Autodesk Inventor part; units mm, degrees
ref_plane "Work Plane2" through (0, 0, 0) normal (0, 0, 1) x (1, 0, 0)
ref_plane "YZ Plane" through (0, 0, 0) normal (1, 0, 0) x (0, 1, 0)
ref_plane "XZ Plane" through (0, 0, 0) normal (0, 1, 0) x (-1, 0, 0)
sketch "Sketch1" plane through (0, 0, 0) normal (0, 0, 1) x (1, 0, 0)
  line L0 (0, 0) -> (114, 0)
  arc A0 (114, 0) -> (114, 18) centre (114, 9) ccw
  arc A1 (0, 21) -> (0, 0) centre (0, 10.5) ccw
  line L1 (0, 21) -> (20.7846, 18)
  line L2 (20.7846, 18) -> (114, 18)
  dimension "d0" = 114
  dimension "d1" = 18
  dimension "d2" = 9
  dimension "d3" = 21
  dimension "d4" = 10.5
  dimension "d5" = 21
extrude "Extrusion1" add sketch "Sketch1" against normal blind 100
sketch "Sketch6" plane through (0, 0, 0) normal (0, 0, 1) x (1, 0, 0)
  line L0 (20.7846, 18) -> (114, 18)
  line L1 (91, 18) -> (114, 18)
  line L2 (114, 18) -> (114, 24)
  line L3 (114, 24) -> (104, 24)
  line L4 (104, 24) -> (100.5359, 22)
  line L5 (100.5359, 22) -> (91, 19)
  line L6 (91, 19) -> (91, 18)
  point P0 (0, 0)
  dimension "d37" = 23
  dimension "d38" = 6
  dimension "d39" = 10
  dimension "d40" = 4
  dimension "d41" = 150
extrude "Extrusion6" add sketch "Sketch6" against normal blind 100
sketch "Sketch7" plane through (0, 0, 0) normal (0, -1, 0) x (1, 0, 0)
  line L0 (0, 0) -> (-10.5, 0)
  line L1 (-10.5, 0) -> (-10.5, -8)
  line L2 (-10.5, 0) -> (-10.5, -100)
  line L3 (-10.5, -8) -> (49, -8)
  line L4 (49, -8) -> (140.4404, 0)
  line L5 (140.4404, 0) -> (-10.5, 0)
  dimension "d44" = 8
  dimension "d45" = 59.5
  dimension "d46" = 90
  dimension "d47" = 175
extrude "Extrusion7" cut sketch "Sketch7" against normal through all
ref_plane "Work Plane2" through (0, 0, 0) normal (0, 0, 1) x (1, 0, 0)
sketch "Sketch8" plane through (0, 0, 0) normal (0, 0, 1) x (1, 0, 0)
  line L0 (-10.5, 0) -> (70, 0)
  line L1 (70, 0) -> (70, 21)
  line L2 (70, 21) -> (-10.5, 21)
  line L3 (-10.5, 21) -> (-10.5, 0)
  line L4 (70, 0) -> (125, 0)
  line L5 (125, 0) -> (125, 18)
  line L6 (125, 18) -> (70, 18)
  line L7 (70, 18) -> (70, 0)
  point P0 (0, 0)
  dimension "d51" = 80.5
  dimension "d52" = 21
  dimension "d53" = 55
  dimension "d54" = 18
extrude "Extrusion8" cut sketch "Sketch8" against normal blind 100
sketch "Sketch9" plane through (91, 18, -100) normal (0, -1, 0) x (1, 0, 0)
  line L0 (23, 97.6868) -> (23, 0)
  line L1 (0, 5) -> (23, 5)
  line L2 (23, 5) -> (23, 7)
  line L3 (23, 7) -> (0, 7)
  line L4 (0, 7) -> (0, 5)
  line L5 (0, 95.6745) -> (0, 0)
  line L6 (0, 23) -> (23, 23)
  line L7 (23, 23) -> (23, 21)
  line L8 (23, 21) -> (0, 21)
  line L9 (0, 21) -> (0, 23)
  line L10 (0, 29) -> (23, 29)
  line L11 (23, 29) -> (23, 31)
  line L12 (23, 31) -> (0, 31)
  line L13 (0, 31) -> (0, 29)
  line L14 (0, 47) -> (23, 47)
  line L15 (23, 47) -> (23, 45)
  line L16 (23, 45) -> (0, 45)
  line L17 (0, 45) -> (0, 47)
  line L18 (0, 53) -> (23, 53)
  line L19 (23, 53) -> (23, 55)
  line L20 (23, 55) -> (0, 55)
  line L21 (0, 55) -> (0, 53)
  line L22 (0, 71) -> (23, 71)
  line L23 (23, 71) -> (23, 69)
  line L24 (23, 69) -> (0, 69)
  line L25 (0, 69) -> (0, 71)
  line L26 (0, 77) -> (23, 77)
  line L27 (23, 77) -> (23, 79)
  line L28 (23, 79) -> (0, 79)
  line L29 (0, 79) -> (0, 77)
  line L30 (0, 89) -> (23, 89)
  line L31 (23, 89) -> (23, 87)
  line L32 (23, 87) -> (0, 87)
  line L33 (0, 87) -> (0, 89)
  point P0 (-91, 100)
  dimension "d57" = 2
  dimension "d58" = 2
  dimension "d59" = 2
  dimension "d60" = 2
  dimension "d61" = 2
  dimension "d62" = 2
  dimension "d63" = 2
  dimension "d64" = 2
extrude "Extrusion9" add sketch "Sketch9" along normal blind 2 contours L0 L32 L5 L30 | L0 L26 L5 L28 | L0 L24 L5 L22 | L0 L18 L5 L20 | L0 L16 L5 L14 | L0 L10 L5 L12 | L0 L8 L5 L6 | L0 L1 L4 L3
sketch "Sketch10" plane through (91, 18, -11) normal (0, -1, 0) x (1, 0, 0)
  circle A0 centre (18, 4) radius 1.5
  circle A1 centre (7, 4) radius 1.5
  circle A2 centre (7, -15) radius 1.5
  circle A3 centre (7, -39) radius 1.5
  circle A4 centre (7, -63) radius 1.5
  circle A5 centre (7, -86.5) radius 1.5
  circle A6 centre (18, -15) radius 1.5
  circle A7 centre (18, -39) radius 1.5
  circle A8 centre (18, -63) radius 1.5
  circle A9 centre (18, -86.5) radius 1.5
  point P0 (-91, 11)
  dimension "d67" = 3
  dimension "d68" = 3
  dimension "d69" = 3
  dimension "d70" = 3
  dimension "d71" = 3
  dimension "d72" = 3
  dimension "d73" = 3
  dimension "d74" = 3
  dimension "d75" = 3
  dimension "d76" = 3
extrude "Extrusion10" cut sketch "Sketch10" against normal through all
fillet "Fillet1" radius 1 7 edges at (114, 24, -51.1566) (109, 24, -100) (102.2679, 23, -100) (95.7679, 20.5, -100) (109, 24, -2.7507) (102.2679, 23, -3.3397) (95.7679, 20.5, -3.9083)
sketch "Sketch12" plane through (91, 18, -93) normal (0, 0, 1) x (1, 0, 0)
  line L0 (23, 0) -> (5, 0)
  line L1 (5, 0) -> (5, 6)
  line L2 (5, 6) -> (23, 6)
  line L3 (23, 6) -> (23, 0)
  point P0 (-91, -18)
  dimension "d84" = 18
  dimension "d85" = 6
extrude "Extrusion12" cut sketch "Sketch12" along normal blind 14
properties part number "Hand - Distal Bridge" material "ABS Plastic"
Model file for the job. Use its own axes, mm. A direction names the side the tool comes from. Coordinates: 2 decimals unless noted, no trailing zeros. Order: outer loops, then holes, each group sorted by start corner. A loop starts at its lowest first (then second) coordinate and runs counter-clockwise, first axis right, second up. Notation, with made-up numbers: (31.5, 64.5) - (87.5, 64.5) arc R6 cw to (87.5, 75.5) - close; hole circle Ø8 at (-15.5, -3.75). An arc over 180 degrees is marked (long way). Return JSON: item names as keys, results as strings. Group by question number.
1) Flat gauge pins, fed straight in: P1, Ø8, axis at x = 96, z = -36, coming from the -Y side; P2, Ø3.5, axis at x = 98, z = -50, coming from the +Y side; P3, Ø4, axis at x = 109, z = -74, coming from the +Y side; P4, Ø0.6, axis at x = 102, y = 17, coming from the -Z side. Where does each tip first touch, or does it go through?
2) Saw through at A-A, the plane z = -41.5. Write the cut outline in (x, y).
3) Mould opens along Z. For faces 4 (the cylindrical face through (102.291, 22.685, -3.609)), 5 (the flat face through (103, 17, -21)), 6 (the flat face through (102, 16, -94)) say: released by +Z, released by -Z, zero draft, split by the parting line, or undercut.
4) Tool access for faces 1 (the cylindrical face through (107.5, 20.96, -6.93)), 2 (the flat face through (102, 17, -53)), 3 (the flat face through (102, 17, -11)): list every direction of +Z, -Z, +X, -X, +Y, -Y with a clear straight run to the whole face (end or side of a thin tool).
5) Probe line 1 (Y direction, x = 107.5, z = -68); line 2 (Z direction, x = 102.5, y = 21.25); line 3 (Z direction, x = 106.5, y = 21). List the from-to ranges inside material, lowest first. Write a range as from..to.
6) Saw through at B-B, the plane z = -7. Write the cut outline in (x, y).
7) Saw through at C-C, the plane x = 98. Count the separate pieces of the cut face and the enclosed holes in it, plus the area to 3 significant figures.
Values found:
{
 "1": {"P1": "stops at y = 18", "P2": "stops at y = 21.75", "P3": "stops at y = 24", "P4": "stops at z = -95"},
 "2": {"outline": "(91, 18) - (114, 18) - (114, 23) arc R1 ccw to (113, 24) - (104, 24) - (100.54, 22) - (91, 19) - close"},
 "3": {"face 4": "released by +Z", "face 5": "undercut", "face 6": "zero draft"},
 "4": {"face 1": "+Y, -Y", "face 2": "+X, -X, -Y", "face 3": "+Z, +X, -X, -Y"},
 "5": {"line 1": "y = 18..24", "line 2": "z = -100..-93, -79..-3.32", "line 3": "z = -100..-93, -79..-2.97"},
 "6": {"outline": "(91, 18) - (96.5, 18) - (96.5, 20.73) - (91, 19) - close; (99.5, 18) - (107.5, 18) - (107.5, 24) - (104, 24) - (100.54, 22) - (99.5, 21.67) - close; (110.5, 18) - (114, 18) - (114, 23) arc R1 ccw to (113, 24) - (110.5, 24) - close"},
 "7": {"separate pieces": "7", "enclosed holes": "0", "area": "247 mm²"}
}
